Check sheet for the modelled part. Datum: model origin and axes. Units: mm. A direction names the side the tool comes from. Round coordinates to 2 decimals unless told otherwise and drop trailing zeros. Write each loop counter-clockwise with the first axis right and the second up, starting at its lowest first coordinate (ties: lowest second). Pieces come first, ordered by that corner, then holes.
from build123d import *

# Parameters (mm, degrees)
F1_DEPTH = 25
F2_W     = 28.4
F2_H     = 25
F3_DEPTH = 5
F5_DEPTH = 28.4


with BuildPart() as f1:
    # F0 (on Top) → F1 (new body)
    with BuildSketch(Plane.XY):
        Polygon((-5.5, 2.5), (-5.5, -12.5), (5.5, -12.5), (5.5, 2.5), (14.2, 2.5), (14.2, 12.5), (-14.2, 12.5), (-14.2, 2.5), align=None)
    extrude(amount=-F1_DEPTH)

    # F2 (on face) → F3 (join)
    with BuildSketch(Plane(origin=(0, 0, -25), x_dir=(1, 0, 0), z_dir=(0, 0, -1))):
        Rectangle(F2_W, F2_H)
    extrude(amount=F3_DEPTH)

    # F4 (on face) → F5 (join)
    with BuildSketch(Plane.YZ.offset(14.2)):
        Polygon((32.5, -64.6410161514), (12.5, -30), (-12.5, -30), (7.5, -64.6410161514), (7.5, -84.6410161514), (32.5, -84.6410161514), align=None)
    extrude(amount=-F5_DEPTH)


solid = f1.part
1. Scan lines: line 1 along Y through (x, z) = (4.5, -13); line 2 along Y through (x, z) = (-9, -22.5); line 3 along X through (y, z) = (-4, -6.5). Record each from-to range of solid material in increasing order.
2. Sectioned sample at B-B, the plane z = -21.5. Enter the section's corners in (x, y), plus the area to 3 significant figures.
3. Go/stop test with flat-tipped pins: pin 1 (12 mm diameter, centred on x = 7.5, z = -10.5, fed in from +Y); pin 2 (6 mm diameter, centred on x = -11, z = -43.5, fed in from -Y); pin 3 (1.5 mm diameter, centred on y = 2, z = -13, fed in from -X); pin 4 (2 mm diameter, centred on x = -6.5, y = -4, fed in from -Z). Record where each tip stops, or that it passes through.
4. Set-up check for faces 1 (the flat face through (10, -5, -25)), 2 (the flat face through (-5.5, -5, -12)), 3 (the flat face through (0, 7.5, -75)): record each of +Z, -Z, +X, -X, +Y, -Y from which the full face is reachable in a straight line by a thin tool's end or side.
5. Sectioned sample at C-C, the plane x = -9.75. Enter the section's corners in (y, z), plus the area to 3 significant figures.
6. Sectioned sample at D-D, the plane y = 22.5. Enter the section's corners in (x, z), plus the area to 3 significant figures.
7. Sectioned sample at A-A, the plane x = -1. Enter the section's corners in (y, z), plus the area to 3 significant figures.
Computed values:
1. line 1: y = -12.5 to 12.5
1. line 2: y = 2.5 to 12.5
1. line 3: x = -5.5 to 5.5
2. outline: (-14.2, 2.5) - (-5.5, 2.5) - (-5.5, -12.5) - (5.5, -12.5) - (5.5, 2.5) - (14.2, 2.5) - (14.2, 12.5) - (-14.2, 12.5) - close
2. area: 449 mm2
3. pin 1: stops at y = 12.5
3. pin 2: stops at y = -6.44
3. pin 3: stops at x = -14.2
3. pin 4: stops at z = -46.45
4. face 1: +Z, +X, -Y
4. face 2: +Z, -X, -Y
4. face 3: -Z, +X, -X, -Y
5. outline: (-12.5, -30) - (7.5, -64.64) - (7.5, -84.64) - (32.5, -84.64) - (32.5, -64.64) - (12.5, -30) - (12.5, 0) - (2.5, 0) - (2.5, -25) - (-12.5, -25) - close
5. area: 1,740 mm2
6. outline: (-14.2, -84.64) - (14.2, -84.64) - (14.2, -47.32) - (-14.2, -47.32) - close
6. area: 1,060 mm2
7. outline: (-12.5, -30) - (7.5, -64.64) - (7.5, -84.64) - (32.5, -84.64) - (32.5, -64.64) - (12.5, -30) - (12.5, 0) - (-12.5, 0) - close
7. area: 2,120 mm2
